Build history of the part. All positions in model axes, mm. A direction names the side the tool comes from. Round coordinates to 2 decimals unless told otherwise and drop trailing zeros. Write each loop counter-clockwise with the first axis right and the second up, starting at its lowest first coordinate (ties: lowest second). Pieces come first, ordered by that corner, then holes. Notation, with made-up numbers: M 15,-38.5 L 21,-38.5 A29 ccw 21,-12.5 Z; hole C -35.75,26 d1. An arc over 180 degrees is marked long. Write item = value, one per line. Start each with the question number.
Q1. Band-saw the part on C-C on z = 139. Write the cut outline in (x, y) (3 decimals).
Q2. Pull direction Y, two halves, no side cores. Call faces 1 (the flat face through (-22.225, -13, 113)), 2 (the flat face through (0, -13, 113)), 3 (the flat face through (-13, -25.4, 113)): released by +Y, released by -Y, zero draft, split by the parting line, or undercut.
Q3. Band-saw the part on D-D on z = 165.1. Write the cut outline in (x, y) (3 decimals).
Q4. Band-saw the part on A-A on z = 209.55. Write the cut outline in (x, y) (3 decimals).
Q5. Probe L1, parallel to X at y = -10.75, z = 116 (3 decimals); L2, parallel to X at y = -0.75, z = 209.55. List the from-to ranges inside material, lowest first.
Q6. Band-saw the part on B-B on y = -10.25. Write the cut outline in (x, z) (3 decimals).
Q7. Tool access for faces 4 (the flat face through (-3.175, -13, 113)), 5 (the cylindrical face through (-13.39, -1.61, 162)): list every direction of +Z, -Z, +X, -X, +Y, -Y with a clear straight run to the whole face (end or side of a thin tool).
Q8. Drop a flat-ended pin along its axis: P1, Ø10, axis at y = -18.5, z = 188, coming from the +X side. Give the stop position or say it passes through.
Autodesk Inventor part; units mm, degrees
ref_plane "YZ Plane" through (0, 0, 0) normal (1, 0, 0) x (0, 1, 0)
ref_plane "XZ Plane" through (0, 0, 0) normal (0, 1, 0) x (-1, 0, 0)
ref_plane "XY Plane" through (0, 0, 0) normal (0, 0, 1) x (1, 0, 0)
sketch "Sketch1" plane through (0, 0, 0) normal (0, 0, 1) x (1, 0, 0)
  line L0 (0, 0) -> (-25.4, 0)
  line L1 (-25.4, 0) -> (-25.4, -25.4)
  line L2 (-25.4, -25.4) -> (0, -25.4)
  line L3 (0, -25.4) -> (0, 0)
  line L4 (-3.175, -22.225) -> (-22.225, -22.225)
  line L5 (-22.225, -22.225) -> (-22.225, -3.175)
  line L6 (-22.225, -3.175) -> (-3.175, -3.175)
  line L7 (-3.175, -3.175) -> (-3.175, -22.225)
  dimension "d0" = 25.4
  dimension "d1" = 25.4
  dimension "d2" = 3.175
extrude "Extrusion1" add sketch "Sketch1" along normal blind 228.6
sketch "Sketch2" plane through (-25.4, -25.4, 0) normal (0, -1, 0) x (1, 0, 0)
  circle A0 centre (12.7, 190.5) radius 4.7625
  line L0 (0, 228.6) -> (25.4, 228.6)
  line L1 (0, 0) -> (0, 228.6)
  circle A1 centre (12.7, 12.7) radius 3.175
  circle A2 centre (14.2875, 58.7375) radius 3.175
  line L2 (0, 0) -> (25.4, 0)
  circle A3 centre (12.7, 209.55) radius 3.3734
  line L3 (25.4, 0) -> (25.4, 228.6)
  circle A4 centre (12.7, 165.1) radius 3.175
  dimension "d5" = 9.525
  dimension "d6" = 38.1
  dimension "d7" = 12.7
  dimension "d10" = 6.35
  dimension "d11" = 12.7
  dimension "d13" = 14.2875
  dimension "d14" = 12.7
  dimension "d15" = 58.7375
  dimension "d16" = 6.7469
  dimension "d17" = 12.7
  dimension "d18" = 19.05
  dimension "d19" = 6.35
  dimension "d20" = 63.5
  dimension "d21" = 12.7
extrude "Extrusion2" cut sketch "Sketch2" against normal blind 152.4 contours A0 | A1 | A2 | A3 | A4
properties part number "15102898-16-A-0205" material "Aluminum 6061"
Conclusion:
q1.outline = M -25.4,-25.4 L 0,-25.4 L 0,0 L -25.4,0 Z; hole M -22.225,-22.225 L -3.175,-22.225 L -3.175,-3.175 L -22.225,-3.175 Z
q2.face_1 = undercut
q2.face_2 = zero draft
q2.face_3 = released by -Y
q3.outline = M -25.4,-25.4 L -15.875,-25.4 L -15.875,-22.225 L -22.225,-22.225 L -22.225,-3.175 L -15.875,-3.175 L -15.875,0 L -25.4,0 Z; M -9.525,-25.4 L 0,-25.4 L 0,0 L -9.525,0 L -9.525,-3.175 L -3.175,-3.175 L -3.175,-22.225 L -9.525,-22.225 Z
q4.outline = M -25.4,-25.4 L -16.073,-25.4 L -16.073,-22.225 L -22.225,-22.225 L -22.225,-3.175 L -16.073,-3.175 L -16.073,0 L -25.4,0 Z; M -9.327,-25.4 L 0,-25.4 L 0,0 L -9.327,0 L -9.327,-3.175 L -3.175,-3.175 L -3.175,-22.225 L -9.327,-22.225 Z
q5.L1 = -25.4 to -22.225, -3.175 to 0
q5.L2 = -25.4 to -16.07, -9.33 to 0
q6.outline = M -25.4,0 L -22.225,0 L -22.225,228.6 L -25.4,228.6 Z; M -3.175,0 L 0,0 L 0,228.6 L -3.175,228.6 Z
q7.face_4 = +Z, -Z
q7.face_5 = +Y, -Y
q8.P1 = 0
